Could you check a few things on this model? Use its own coordinates, in mm. A direction names the side the tool comes from. Give positions to 0.01 mm unless a question says otherwise; leave off trailing zeros. Loops run counter-clockwise (first coordinate to the right, second up) from the corner with the lowest first, then second, coordinate; pieces in that order, holes last. Notation, with made-up numbers: (-0.75, 65.25) - (50.25, 65.25) arc R16 ccw to (50.25, 93.25) - close; hole circle Ø4 at (-7, -11.5). An arc over 180 degrees is marked (long way). One line per item, written item: value. Start each with the question number.
Q1. I want a section at B-B (x = -508). Please give me the cut outline in (y, z).
Q2. I'm going to push flat-ended pins straight in: P1, Ø1.5, axis at x = 105.5, z = 1, coming from the -Y side; P2, Ø1.5, axis at x = 803.5, z = 3, coming from the -Y side; P3, Ø1.5, axis at x = -49.5, z = 4, coming from the -Y side. Where does each tip first touch, or does it pass through?
Q3. If we mould it in two halves opening along Y, with no side actions, what happens to faces 1 (the face through (-265.45, -1.85, 2.35)), 2 (the face through (1043.45, -2.16, 2.35)), 3 (the face through (829.693, -1.445, 2.348))? For each: released by +Y, released by -Y, zero draft, split by the parting line, or undercut.
Q4. I want a section at A-A (y = 95.5). Count the separate pieces of the cut face and the enclosed holes in it, then the cut area to 3 significant figures.
Q5. If I drill on line 1 (Y direction, x = -546.5, z = 0.6); line 2 (Y direction, x = -257.5, z = 1.65), over which ranges is the centre line in solid material (lowest first)? Write a range as from..to.
Q6. For faces 4 (the face through (-815.486, -2.228, 2.348)), 5 (the face through (464.8, -1.85, 2.35)), 6 (the face through (284, 11, 4.762)), which set-ups out of +Z, -Z, +X, -X, +Y, -Y let a thin tool reach every point of the face, with its end or its side?
```python
from build123d import *

# Parameters (mm, degrees)
F0_W     = 12.7
F0_H     = 0.254
F0_H_2   = 291.084
F0_W_2   = 9.525
F1_DEPTH = 4.7625


# Not quite as in the source:
# - a feature names something its author has since deleted; it is built from what else it names


with BuildPart() as f1:
    # F0 (on Top) → F1 (new body)
    with BuildSketch(Plane.XY):
        Polygon((-1095.375, 145.669), (-1168.4, 145.669), (-1168.4, 145.415), (-1095.2286143575, 145.415), align=None)
        with Locations((-1174.75, 145.542)):
            Rectangle(F0_W, F0_H)
        with Locations((-1174.75, -0.127)):
            Rectangle(F0_W, F0_H_2)
        with BuildLine():
            Line((1001.7125, 145.669), (935.0375, 145.669))
            Line((935.0375, 145.669), (935.0375, -145.669))
            Line((935.0375, -145.669), (971.4705200239, -145.669))
            Line((971.4705200239, -145.669), (1117.4725985353, 145.415))
            Line((1117.4725985353, 145.415), (1117.6, 145.669))
            Line((1117.6, 145.669), (1103.3919799761, 145.669))
            Line((1103.3919799761, 145.669), (957.9830261901, -144.232488632))
            ThreePointArc((957.9830261901, -144.232488632), (957.67894626, -144.3606444457), (957.5048911047, -144.080299445))
            Line((957.5048911047, -144.080299445), (1001.7125, 145.669))
        make_face()
        with BuildLine():
            Line((-1080.7168319418, 145.669), (-1095.375, 145.669))
            Line((-1095.375, 145.669), (-1095.2286143575, 145.415))
            Line((-1095.2286143575, 145.415), (-927.4706680582, -145.669))
            Line((-927.4706680582, -145.669), (-898.1543319418, -145.669))
            Line((-898.1543319418, -145.669), (-730.4700684279, 145.2871498423))
            ThreePointArc((-730.4700684279, 145.2871498423), (-730.25, 145.4143196918), (-730.0299315721, 145.2871498423))
            Line((-730.0299315721, 145.2871498423), (-562.3456680582, -145.669))
            Line((-562.3456680582, -145.669), (-533.0293319418, -145.669))
            Line((-533.0293319418, -145.669), (-365.3450684279, 145.2871498423))
            ThreePointArc((-365.3450684279, 145.2871498423), (-365.125, 145.4143196918), (-364.9049315721, 145.2871498423))
            Line((-364.9049315721, 145.2871498423), (-197.2206680582, -145.669))
            Line((-197.2206680582, -145.669), (-167.9043319418, -145.669))
            Line((-167.9043319418, -145.669), (-0.2200684279, 145.2871498423))
            ThreePointArc((-0.2200684279, 145.2871498423), (0, 145.4143196918), (0.2200684279, 145.2871498423))
            Line((0.2200684279, 145.2871498423), (167.9043319418, -145.669))
            Line((167.9043319418, -145.669), (197.2206680582, -145.669))
            Line((197.2206680582, -145.669), (364.9049315721, 145.2871498423))
            ThreePointArc((364.9049315721, 145.2871498423), (365.125, 145.4143196918), (365.3450684279, 145.2871498423))
            Line((365.3450684279, 145.2871498423), (533.0293319418, -145.669))
            Line((533.0293319418, -145.669), (562.3456680582, -145.669))
            Line((562.3456680582, -145.669), (730.0299315721, 145.2871498423))
            ThreePointArc((730.0299315721, 145.2871498423), (730.25, 145.4143196918), (730.4700684279, 145.2871498423))
            Line((730.4700684279, 145.2871498423), (898.1543319418, -145.669))
            Line((898.1543319418, -145.669), (935.0375, -145.669))
            Line((935.0375, -145.669), (935.0375, 145.669))
            Line((935.0375, 145.669), (868.3625, 145.669))
            Line((868.3625, 145.669), (912.6085893136, -144.3325111014))
            ThreePointArc((912.6085893136, -144.3325111014), (912.4415096754, -144.6105240597), (912.137426584, -144.4976511932))
            Line((912.137426584, -144.4976511932), (744.9081680582, 145.669))
            Line((744.9081680582, 145.669), (715.5918319418, 145.669))
            Line((715.5918319418, 145.669), (547.9075684279, -145.2871498423))
            ThreePointArc((547.9075684279, -145.2871498423), (547.6875, -145.4143196918), (547.4674315721, -145.2871498423))
            Line((547.4674315721, -145.2871498423), (379.7831680582, 145.669))
            Line((379.7831680582, 145.669), (350.4668319418, 145.669))
            Line((350.4668319418, 145.669), (182.7825684279, -145.2871498423))
            ThreePointArc((182.7825684279, -145.2871498423), (182.5625, -145.4143196918), (182.3424315721, -145.2871498423))
            Line((182.3424315721, -145.2871498423), (14.6581680582, 145.669))
            Line((14.6581680582, 145.669), (-14.6581680582, 145.669))
            Line((-14.6581680582, 145.669), (-182.3424315721, -145.2871498423))
            ThreePointArc((-182.3424315721, -145.2871498423), (-182.5625, -145.4143196918), (-182.7825684279, -145.2871498423))
            Line((-182.7825684279, -145.2871498423), (-350.4668319418, 145.669))
            Line((-350.4668319418, 145.669), (-379.7831680582, 145.669))
            Line((-379.7831680582, 145.669), (-547.4674315721, -145.2871498423))
            ThreePointArc((-547.4674315721, -145.2871498423), (-547.6875, -145.4143196918), (-547.9075684279, -145.2871498423))
            Line((-547.9075684279, -145.2871498423), (-715.5918319418, 145.669))
            Line((-715.5918319418, 145.669), (-744.9081680582, 145.669))
            Line((-744.9081680582, 145.669), (-912.5924315721, -145.2871498423))
            ThreePointArc((-912.5924315721, -145.2871498423), (-912.8125, -145.4143196918), (-913.0325684279, -145.2871498423))
            Line((-913.0325684279, -145.2871498423), (-1080.7168319418, 145.669))
        make_face()
        Polygon((1212.85, 145.415), (1212.85, -145.669), (1225.55, -145.669), (1225.55, 145.669), (1212.85, 145.669), align=None)
        Polygon((1117.6, 145.669), (1117.4725985353, 145.415), (1203.325, 145.415), (1203.325, 145.669), align=None)
        with Locations((1208.0875, 145.542)):
            Rectangle(F0_W_2, F0_H)
    extrude(amount=F1_DEPTH)


solid = f1.part
```
Worked answers:
1. outline: (-102.24, 0) - (-76.81, 0) - (-76.81, 4.76) - (-102.24, 4.76) - close
2. P1: stops at y = -38.69
2. P2: stops at y = 17.27
2. P3: stops at y = 58.48
3. face 1: released by +Y
3. face 2: released by -Y
3. face 3: undercut
4. separate pieces: 15
4. enclosed holes: 0
4. area: 1,520 mm²
5. line 1: y = -145.67..-143.61
5. line 2: y = -41.08..-15.64
6. face 4: +Z, -Z, -Y
6. face 5: +Z, -Z, +Y
6. face 6: +Z, +X, -X, +Y, -Y
